Read the model definition and answer for the solid it produces. Units are mm, in the model's axes. A direction names the side the tool comes from. Round coordinates to 2 decimals unless told otherwise and drop trailing zeros. Loops run counter-clockwise (first coordinate to the right, second up) from the corner with the lowest first, then second, coordinate; pieces in that order, holes last. Notation, with made-up numbers: (82, 49.25) -> (96, 49.25) arc R20 cw to (96, 85.25) -> close; hole circle Ø9 at (-1, 6). An arc over 180 degrees is marked (long way). Put each result on its own line as item: value.
from build123d import *
from build123d import SkipClean  # not in build123d's __all__

# Parameters (mm, degrees)
F0_R      = 14.5
F1_DEPTH  = 40
F2_R      = 5
F3_R      = 5
F4_W      = 15
F4_H      = 15
F4_R      = 3
F5_DEPTH  = 25
F6_W      = 110.2663613856
F6_H      = 71.1540803313
F7_DEPTH  = 50.001
F9_W      = 49.9149149903
F9_H      = 20
F10_DEPTH = 28.501


with BuildPart() as f1:
    # F0 (on Front) → F1 (new body)
    with BuildSketch(Plane.XZ):
        with BuildLine():
            Line((-13.6106575888, -11), (-50, -11))
            Line((-50, -11), (-50, -16))
            Line((-50, -16), (50, -16))
            Line((50, -16), (50, -11))
            Line((50, -11), (13.6106575888, -11))
            ThreePointArc((13.6106575888, -11), (0, 17.5), (-13.6106575888, -11))
        make_face()
        Circle(F0_R, mode=Mode.SUBTRACT)
    extrude(amount=F1_DEPTH)

    # F2
    f2_edges = [f1.edges().sort_by_distance(p)[0] for p in [
        (13.610658, -20, -11),
        (-13.610658, -20, -11),
    ]]
    fillet(f2_edges, radius=F2_R)

    # F3
    f3_edges = [f1.edges().sort_by_distance(p)[0] for p in [
        (50, -40, -13.5),
        (-50, -40, -13.5),
        (50, 0, -13.5),
        (-50, 0, -13.5),
    ]]
    fillet(f3_edges, radius=F3_R)

    # F4 (on face) → F5 (cut)
    with BuildSketch(Plane.XY.offset(-11)):
        with Locations((-35.6688876305, -17.775596238)):
            Rectangle(F4_W, F4_H)
        with Locations((-45, -35)):
            Circle(F4_R)
        with Locations((-28.1688876305, -35.0887903643)):
            Circle(F4_R)
        with Locations((-45, -5)):
            Circle(F4_R)
        with Locations((-27.3576099426, -5)):
            Circle(F4_R)
    extrude(amount=-F5_DEPTH, mode=Mode.SUBTRACT)

    # F6 (on Right) → F7 (cut, through all)
    with BuildSketch(Plane.YZ):
        with Locations((-21.3294159621, -6.3556879759)):
            Rectangle(F6_W, F6_H)
    extrude(amount=F7_DEPTH, mode=Mode.SUBTRACT)

    # F8: F1 across plane


with BuildPart() as f1_1:
    add(f1.part, clean=False)
    with SkipClean():  # cleaning this boolean's faces spoils the solid; the shape is the same uncleaned
        add(f1.part.mirror(Plane.YZ), clean=False)

    # F9 (on face) → F10 (cut, through all)
    with BuildSketch(Plane.XY.offset(-11)):
        Polygon((-21.6852484422, -10), (-31.6722874067, -10), (-31.6722874067, -10.275596238), (-28.1688876305, -10.275596238), (-28.1688876305, -25.275596238), (-31.6722874067, -25.275596238), (-31.6722874067, -30), (-21.6852484422, -30), align=None)
        with Locations((3.272209053, -20)):
            Rectangle(F9_W, F9_H)
    with SkipClean():  # cleaning this boolean's faces spoils the solid; the shape is the same uncleaned
        extrude(amount=F10_DEPTH, mode=Mode.SUBTRACT)


solid = f1_1.part
Item 1: The part is cut by section C-C (x = 1). Determine the outline of the cut face in (y, z).
Derived:
outline: (-40, -16) -> (0, -16) -> (0, -14.47) -> (-40, -14.47) -> close; (-40, 14.47) -> (-30, 14.47) -> (-30, 17.47) -> (-40, 17.47) -> close; (-10, 14.47) -> (0, 14.47) -> (0, 17.47) -> (-10, 17.47) -> close
Item 2: Which of the six approach directions +Z, -Z, +X, -X, +Y, -Y give full straight-line access (tool end or side, diameter ignored) to faces 3 (the flat face through (-43.169, -18, -13)), 4 (the flat face through (-5, -30, 14)), 5 (the cylindrical face through (-49, -38, -14))?
Derived:
face 3: +Z, -Z
face 4: +Z, +X, -X
face 5: +Z, -Z, -X, -Y
Item 3: Flat-ended cylindrical pins translate along their axes: pin 1 Ø9.5 at (x, y) = (45, -35) entering from -Z; pin 2 Ø8 at (y, z) = (-6.5, 4) entering from -X; pin 3 Ø22.5 at (x, y) = (-36, -28) entering from +Z; pin 4 Ø3 at (y, z) = (-35.5, 10) entering from -X. Find the tip coordinate at first contact, or state that the pin passes through.
Derived:
pin 1: stops at z = -16
pin 2: stops at x = -17.5
pin 3: stops at z = -11
pin 4: stops at x = -15.3
Item 4: The part is cut by section A-A (y = -21). Determine the outline of the cut face in (x, z).
Derived:
outline: (-50, -16) -> (-43.17, -16) -> (-43.17, -11) -> (-50, -11) -> close; (-28.17, -16) -> (28.17, -16) -> (28.17, -11) -> (9.45, -11) arc R14.5 cw to (-9.45, -11) -> (-28.17, -11) -> close; (43.17, -16) -> (50, -16) -> (50, -11) -> (43.17, -11) -> close
Item 5: For a pull along Z with two mould halves and no side action, classify faces 1 (the cylindrical face through (-17.745, -5.07, -9.079)), 2 (the cylindrical face through (49, -38, -14)) as pulls with the +Z half, pulls with the -Z half, needs draft (parallel to the pull), parting line crosses it, or undercut.
Derived:
face 1: undercut
face 2: needs draft
Item 6: Find the intervals of material crossed by line 1 along Y through (x, z) = (-45, -12.45); line 2 along Y through (x, z) = (7.5, 15); line 3 along Z through (x, y) = (-34, -4), in increasing order.
Derived:
line 1: y = -40 to -38, -32 to -8, -2 to 0
line 2: y = -40 to -30, -10 to 0
line 3: z = -16 to -11
Item 7: The part is cut by section D-D (z = -12). State how many separate pieces and enclosed holes the cut face has, then the cut area to 3 significant figures.
Derived:
separate pieces: 2
enclosed holes: 10
area: 2,650 mm^2
Item 8: The part is cut by section B-B (z = 0). Determine the outline of the cut face in (x, y), then the cut area to 3 significant figures.
Derived:
outline: (-17.5, -40) -> (-14.5, -40) -> (-14.5, -30) -> (-17.5, -30) -> close; (-17.5, -10) -> (-14.5, -10) -> (-14.5, 0) -> (-17.5, 0) -> close; (14.5, -40) -> (17.5, -40) -> (17.5, -30) -> (14.5, -30) -> close; (14.5, -10) -> (17.5, -10) -> (17.5, 0) -> (14.5, 0) -> close
area: 120 mm^2
